Work out the finished part from the listing and answer in its coordinate system (mm). A direction names the side the tool comes from. Coordinates: 2 decimals unless noted, no trailing zeros. Order: outer loops, then holes, each group sorted by start corner. A loop starts at its lowest first (then second) coordinate and runs counter-clockwise, first axis right, second up. Notation, with made-up numbers: M 29.25,70.25 L 51.25,70.25 A17 ccw 51.25,89.25 Z; hole C 16,-37 d5. An arc over 180 degrees is marked long. Answer in a Markdown table with one row per item. Add a question column.
Item 1: The part is cut by section A-A (x = 0). Write down the section's boundary in (y, z).
Item 2: The mould has two halves that part along X. Classify faces 1 (the face through (-83, 18, 0)), 2 (the face through (72, 16, 0)), 3 (the face through (69.153, 8.252, 0.35)), 4 (the face through (-105.64, 15.21, 9.1)): released by +X, released by -X, zero draft, split by the parting line, or undercut.
Item 3: Flat-ended cylindrical pins translate along their axes: pin 1 Ø1.7 at (x, z) = (-79.25, -7) entering from +Y; pin 2 Ø1 at (y, z) = (6, 1) entering from -X; pin 3 Ø2 at (y, z) = (5.5, -17.5) entering from +X; pin 4 Ø1.1 at (x, z) = (77, -1.5) entering from -Y. Find the tip coordinate at first contact, or state that the pin passes through.
Item 4: The part is cut by section C-C (z = 0). State how many separate pieces and enclosed holes the cut face has, then the cut area to 3 significant figures.
Item 5: The part is cut by section D-D (x = -49). Write down the section's boundary in (y, z), then the cut area to 3 significant figures.
Item 6: Consider line 1 (X direction, y = 17, z = 7); line 2 (X direction, y = 13.5, z = -20); line 3 (X direction, y = 14.5, z = -7). Determine where each line is inside the solid, lowest interval first. Write a range as from..to.
Item 7: Which of the six approach directions +Z, -Z, +X, -X, +Y, -Y give full straight-line access (tool end or side, diameter ignored) to faces 5 (the face through (77, 5.6, 0)), 6 (the face through (15, 2, 0)), 7 (the face through (-76.97, 16.75, 17.6)), 8 (the face through (76.822, 10.586, 0.35))?
from build123d import *

# Parameters (mm, degrees)
BOSS_EXTRUDE1_DEPTH     = 25
SKETCH2_R               = 14.25
CUT_EXTRUDE1_DEPTH      = 50
CUT_EXTRUDE1_DRAFT      = -3
CUT_EXTRUDE2_DEPTH      = 85.581854283
REVOLVE1_ANGLE          = 30
FILLET1_R               = 0.2
FILLET4_R               = 1
BOSS_EXTRUDE2_START     = -25
BOSS_EXTRUDE2_DEPTH     = 50
FILLET5_R               = 0.5
BOSS_EXTRUDE3_DEPTH     = 10
SKETCH7_R               = 1.45
CUT_EXTRUDE3_DEPTH      = 111.865909999
BOSS_EXTRUDE5_START     = 2
SKETCH9_R               = 3
SKETCH9_R_2             = 1.45
BOSS_EXTRUDE5_DEPTH     = 2
FILLET6_R               = 3
CUT_EXTRUDE4_DEPTH      = 112.208138191
CUT_EXTRUDE4_DEPTH_BACK = 112.208138191
SKETCH10_W              = 29.886864559
SKETCH10_H              = 5.5


with BuildPart() as part:
    # Sketch1 → Boss-Extrude1 (new, symmetric)
    with BuildSketch(Plane.XY):
        with BuildLine():
            Line((0, 0), (-68.25, 0))
            Line((-68.25, 0), (-70, 16))
            Line((-70, 16), (-73.75, 16))
            ThreePointArc((-73.75, 16), (-75.596738759, 15.293339066), (-76.5, 13.534381178))
            Line((-76.5, 13.534381178), (-77.214697941, 7))
            Line((-77.214697941, 7), (-79.202841325, 7.217453183))
            Line((-79.202841325, 7.217453183), (-78.488143384, 13.75183436))
            ThreePointArc((-78.488143384, 13.75183436), (-76.931859285, 16.782450607), (-73.75, 18))
            Line((-73.75, 18), (-68.206822675, 18))
            Line((-68.206822675, 18), (-66.456822675, 2))
            Line((-66.456822675, 2), (0, 2))
            Line((0, 2), (0, 0))
        make_face()
    boss_extrude1 = extrude(amount=BOSS_EXTRUDE1_DEPTH, both=True)

    # Mirror1: Boss-Extrude1 across plane
    add(boss_extrude1.mirror(Plane(origin=(0, 0, 25), x_dir=(0, 0, 1), z_dir=(-1, 0, 0))))


with BuildPart() as cut_extrude1_tool:
    # Sketch2 → Cut-Extrude1 (with draft: the straight prism first)
    with BuildSketch(Plane(origin=(0, 2, 0), x_dir=(1, 0, 0), z_dir=(0, 1, 0))):
        Circle(SKETCH2_R)
    extrude(amount=-CUT_EXTRUDE1_DEPTH)
    # Cut-Extrude1: the draft: its side faces are tilted about the plane it starts from
    cut_extrude1_sides = [cut_extrude1_tool.faces().sort_by_distance(p)[0] for p in [
        (-14.25, -23, 0),
    ]]
    draft(cut_extrude1_sides, Plane(origin=(0, 2, 0), x_dir=(1, 0, 0), z_dir=(0, 1, 0)), CUT_EXTRUDE1_DRAFT)


with BuildPart() as part_1:
    add(part.part)

    # Cut-Extrude1: cut by cut_extrude1_tool
    add(cut_extrude1_tool.part, mode=Mode.SUBTRACT)

    # Sketch3 → Cut-Extrude2 (cut, through all)
    with BuildSketch(Plane(origin=(0, 2, 0), x_dir=(1, 0, 0), z_dir=(0, 1, 0))):
        with BuildLine():
            Line((-18.75, 8.25), (-18.75, -8.25))
            Line((-18.75, -8.25), (-13.854714901, -8.25))
            ThreePointArc((-13.854714901, -8.25), (-16.125, 0), (-13.854714901, 8.25))
            Line((-13.854714901, 8.25), (-18.75, 8.25))
        make_face()
        with BuildLine():
            Line((18.75, 8.25), (18.75, -8.25))
            Line((18.75, -8.25), (13.854714901, -8.25))
            ThreePointArc((13.854714901, -8.25), (16.125, 0), (13.854714901, 8.25))
            Line((13.854714901, 8.25), (18.75, 8.25))
        make_face()
    extrude(amount=-CUT_EXTRUDE2_DEPTH, mode=Mode.SUBTRACT)

    # Sketch4 → Revolve1 (revolve, symmetric)
    with BuildSketch(Plane.XY) as revolve1_sk:
        with BuildLine():
            Line((16.125, 0), (16.125, 2))
            ThreePointArc((16.125, 2), (17, 1), (16.125, 0))
        make_face()
    revolve1 = revolve(axis=Axis((0, 2, 0), (0, 1, 0)), revolution_arc=REVOLVE1_ANGLE / 2)
    revolve1 = revolve1 + revolve(revolve1_sk.sketch, axis=Axis((0, 2, 0), (0, -1, 0)), revolution_arc=REVOLVE1_ANGLE / 2)

    # Mirror2: Revolve1 across plane
    add(revolve1.mirror(Plane(origin=(0, 0, 0), x_dir=(0, 0, 1), z_dir=(1, 0, 0))))

    # Fillet1
    fillet1_edges = [part_1.edges().sort_by_distance(p)[0] for p in [
        (-70, 16, 0),
        (70, 16, 0),
    ]]
    fillet(fillet1_edges, radius=FILLET1_R)

    # Fillet4
    fillet4_edges = [part_1.edges().sort_by_distance(p)[0] for p in [
        (-68.25, 0, 0),
        (-68.206822675, 18, 0),
        (-66.456822675, 2, 0),
        (68.25, 0, 0),
        (68.206822675, 18, 0),
        (66.456822675, 2, 0),
    ]]
    fillet(fillet4_edges, radius=FILLET4_R)

    # Sketch6 → Boss-Extrude2 (add)
    with BuildSketch(Plane.XY.offset(BOSS_EXTRUDE2_START)):
        Polygon((79.226625267, 7), (79.226625267, 5.6), (75.714697941, 5.6), (75.714697941, 7), (77.214697941, 7), (79.202841325, 7.217453183), align=None)
    extrude(amount=BOSS_EXTRUDE2_DEPTH)

    # Fillet5
    fillet5_edges = [part_1.edges().sort_by_distance(p)[0] for p in [
        (75.714697941, 7, 0),
        (77.214697941, 7, 0),
    ]]
    fillet(fillet5_edges, radius=FILLET5_R)

    # Sketch5 → Boss-Extrude3 (add, symmetric)
    with BuildSketch(Plane.XY):
        with BuildLine():
            Line((-73.75, 18), (-106.5, 18))
            Line((-106.5, 18), (-106.5, 7))
            Line((-106.5, 7), (-77.214697941, 7))
            Line((-77.214697941, 7), (-76.5, 13.534381178))
            ThreePointArc((-76.5, 13.534381178), (-75.596738759, 15.293339066), (-73.75, 16))
            Line((-73.75, 16), (-73.75, 18))
        make_face()
    extrude(amount=BOSS_EXTRUDE3_DEPTH, both=True)

    # Sketch7 → Cut-Extrude3 (cut, through all)
    with BuildSketch(Plane(origin=(0, 18, 0), x_dir=(1, 0, 0), z_dir=(0, 1, 0))):
        with Locations(Location((-79.25, 7, 0), (0, 0, 270))):
            Circle(SKETCH7_R)
        with Locations(Location((-103.5, -7, 0), (0, 0, 270))):
            Circle(SKETCH7_R)
    extrude(amount=-CUT_EXTRUDE3_DEPTH, mode=Mode.SUBTRACT)

    # Sketch9 → Boss-Extrude5 (add)
    # profile 1 of 2: a face of its own
    with BuildSketch(Plane(origin=(0, 18, 0), x_dir=(1, 0, 0), z_dir=(0, 1, 0)).offset(BOSS_EXTRUDE5_START)):
        with Locations(Location((-79.25, 7, 0), (0, 0, 90))):
            Circle(SKETCH9_R)
        with Locations(Location((-79.25, 7, 0), (0, 0, 270))):
            Circle(SKETCH9_R_2, mode=Mode.SUBTRACT)
    # profile 2 of 2: a face of its own
    with BuildSketch(Plane(origin=(0, 18, 0), x_dir=(1, 0, 0), z_dir=(0, 1, 0)).offset(BOSS_EXTRUDE5_START)):
        with Locations(Location((-103.5, -7, 0), (0, 0, 270))):
            Circle(SKETCH9_R)
        with Locations(Location((-103.5, -7, 0), (0, 0, 270))):
            Circle(SKETCH9_R_2, mode=Mode.SUBTRACT)
    extrude(amount=-BOSS_EXTRUDE5_DEPTH)

    # Fillet6
    fillet6_edges = [part_1.edges().sort_by_distance(p)[0] for p in [
        (-106.5, 12.5, 10),
        (-106.5, 12.5, -10),
    ]]
    fillet(fillet6_edges, radius=FILLET6_R - 0.0001)  # a hair under: the kernel refuses the full size

    # Sketch10 → Cut-Extrude4 (cut, two sides: drawn at the far end of the back side and taken through both)
    with BuildSketch(Plane.XY.offset(-CUT_EXTRUDE4_DEPTH_BACK)):
        with Locations((-91.55656772, 9.75)):
            Rectangle(SKETCH10_W, SKETCH10_H)
    extrude(amount=CUT_EXTRUDE4_DEPTH + CUT_EXTRUDE4_DEPTH_BACK, mode=Mode.SUBTRACT)


solid = part_1.part
Reply:
| question | item | result |
|---|---|---|
| 1 | outline | M 0,-25 L 2,-25 L 2,-14.25 L 0,-14.15 Z; M 0,14.15 L 2,14.25 L 2,25 L 0,25 Z |
| 2 | face 1 | zero draft |
| 2 | face 2 | undercut |
| 2 | face 3 | undercut |
| 2 | face 4 | released by -X |
| 3 | pin 1 | passes through |
| 3 | pin 2 | stops at x = -68.96 |
| 3 | pin 3 | stops at x = 79.23 |
| 3 | pin 4 | stops at y = 5.6 |
| 4 | separate pieces | 4 |
| 4 | enclosed holes | 0 |
| 4 | area | 489 mm2 |
| 5 | outline | M 0,-25 L 2,-25 L 2,25 L 0,25 Z |
| 5 | area | 100 mm2 |
| 6 | line 1 | x = -106.5..-104.95, -102.05..-68.1, 68.1..76.67 |
| 6 | line 2 | x = -78.52..-76.5, -69.73..-67.71, 67.71..69.73, 76.5..78.52 |
| 6 | line 3 | x = -106.5..-80.7, -77.8..-76.21, -69.84..-67.82, 67.82..69.84, 76.21..78.35 |
| 7 | face 5 | +Z, -Z, +X, -Y |
| 7 | face 6 | +Z, -Z, +Y |
| 7 | face 7 | +Z, -X, +Y |
| 7 | face 8 | +Z, -Z |
